from build123d import *

# Parameters (mm, degrees)
PAD003_DEPTH         = 6.35
SKETCH015_R          = 1.524
POCKET003_DEPTH      = 4.7635
POCKET003_DEPTH_BACK = 1.5885
SKETCH016_W          = 3.175
SKETCH016_H          = 12.7
PAD008_DEPTH         = 67.7
SKETCH025_W          = 28.575
SKETCH025_H          = 24.775
PAD009_DEPTH         = 3.175
POCKET007_DEPTH      = 5.175996
PAD010_DEPTH         = 3.175
CHAMFER001_SIZE      = 3.1496


with BuildPart() as part:
    # Sketch014 → Pad003 (new body, symmetric)
    with BuildSketch(Plane.YZ.offset(15.25)):
        with BuildLine():
            ThreePointArc((-1.430625, 0), (0.315625, -1.74625), (2.061875, 0))
            Line((2.061875, 5.63), (2.061875, 0))
            ThreePointArc((3.490625, 4.20125), (3.072154, 5.211529), (2.061875, 5.63))
            Line((3.490625, 4.20125), (3.490625, 0))
            ThreePointArc((0.315625, -3.175), (2.560689, -2.245064), (3.490625, 0))
            Line((-2.859375, -3.175), (0.315625, -3.175))
            Line((-2.859375, 4.20125), (-2.859375, -3.175))
            ThreePointArc((-1.430625, 5.63), (-2.440904, 5.211529), (-2.859375, 4.20125))
            Line((-1.430625, 5.63), (-1.430625, 0))
        make_face()
    extrude(amount=PAD003_DEPTH, both=True)

    # Sketch015 (on Face72 of LinearPattern001) → Pocket003 (cut, two sides)
    with BuildSketch(Plane.XZ.offset(1.271875)) as pocket003_sk:
        with Locations((12.075, 2.815)):
            Circle(SKETCH015_R)
        with Locations((18.425, 2.815)):
            Circle(SKETCH015_R)
    extrude(amount=-POCKET003_DEPTH, mode=Mode.SUBTRACT)
    extrude(pocket003_sk.sketch, amount=POCKET003_DEPTH_BACK, mode=Mode.SUBTRACT)

    # Sketch016 (on Face8 of Pocket003) → Pad008 (join)
    with BuildSketch(Plane(origin=(15.25, -2.859375, 0), x_dir=(0, 0, -1), z_dir=(0, -1, 0))):
        with Locations((1.5875, 0)):
            Rectangle(SKETCH016_W, SKETCH016_H)
    extrude(amount=PAD008_DEPTH)

    # Sketch025 (on Face16 of Pad008) → Pad009 (join)
    with BuildSketch(Plane(origin=(15.25, 0, 0), x_dir=(0, -1, 0), z_dir=(0, 0, 1))):
        with Locations((56.271875, -18.7375)):
            Rectangle(SKETCH025_W, SKETCH025_H)
    extrude(amount=-PAD009_DEPTH)

    # Sketch026 (on Face29 of Pad015) → Pocket007 (cut, through all)
    with BuildSketch(Plane(origin=(15.25, 0, 1.999996), x_dir=(0, -1, 0), z_dir=(0, 0, 1))):
        with BuildLine():
            ThreePointArc((61.161375, -8.9), (57.859375, -5.598), (54.557375, -8.9))
            Line((54.557375, -8.9), (54.557375, -21.6))
            ThreePointArc((54.557375, -21.6), (57.859375, -24.902), (61.161375, -21.6))
            Line((61.161375, -21.6), (61.161375, -8.9))
        make_face()
    extrude(amount=-POCKET007_DEPTH, mode=Mode.SUBTRACT)

    # Sketch027 (on Face24 of Pocket007) → Pad010 (join)
    with BuildSketch(Plane(origin=(15.25, 0, -3.175), x_dir=(0, 1, 0), z_dir=(0, 0, -1))):
        Polygon((-2.859375, 6.35), (-45.159375, 6.35), (-45.159375, -31.125), (-41.984375, -31.125), (-41.984375, 3.175), (-2.859375, 3.175), align=None)
    extrude(amount=PAD010_DEPTH)

    # Chamfer001
    chamfer001_edges = [part.edges().sort_by_distance(p)[0] for p in [
        (20.0125, -2.859375, -6.35),
        (-15.875, -43.571875, -6.35),
    ]]
    chamfer(chamfer001_edges, length=CHAMFER001_SIZE)


solid = part.part
Part model, mm, in its own coordinate system. A direction names the side the tool comes from. Coordinates: 2 decimals unless noted, no trailing zeros. Loops run counter-clockwise (first coordinate to the right, second up) from the corner with the lowest first, then second, coordinate; pieces in that order, holes last. Notation, with made-up numbers: (-30, 65.5) -> (13, 65.5) arc R24 cw to (13, 82.5) -> close; hole circle Ø6 at (-21, 69). An arc over 180 degrees is marked (long way). Use a Markdown table: item, result. Add a question column.
Item 1: Band-saw the part on A-A on x = -4.5. Write the cut outline in (y, z) (3 decimals).
Item 2: Probe probe 1 along Y at (x, z) = (-5, -2.5); probe 2 along Y at (x, z) = (-13.5, -0.5); probe 3 along X at (y, z) = (-60, -2.5) (3 decimals). List the from-to ranges inside material, lowest first.
Item 3: Which spindle directions (+Z, -Z, +X, -X, +Y, -Y) get a long thin tool onto all of the face, cutting with end or side? Do faces 5 (the flat face through (3, -52, -3.175)), 6 (the flat face through (15, 2.062, 3)), 7 (the flat face through (8.9, -17, -2)), 8 (the flat face through (0, -54.557, -2)), 9 (the flat face through (7, -44, 0)). Say none if no direction does.
Item 4: Band-saw the part on C-C on x = -12. Write the cut outline in (y, z) (3 decimals), plus the area to 3 significant figures.
Item 5: Pull direction Y, two halves, no side cores. Call faces 1 (the flat face through (15, -2.859, 2)), 2 (the flat face through (19.99, -4.41, -4.75)), 3 (the flat face through (14, -21, -3.175)), 4 (the flat face through (15, -1.431, 3)): +Y half, -Y half, draft (parallel to the pull), parting line (faces both ways), or undercut.
Item 6: Band-saw the part on B-B on z = -2.5. Write the cut outline in (x, y) (3 decimals).
Item 7: Flat gauge pins, fed straight in: P1, Ø3.5, axis at y = -24, z = -5, coming from the -X side (3 decimals); P2, Ø1, axis at x = 1.5, z = -1, coming from the +Y side; P3, Ø5, axis at x = 1, z = 1.5, coming from the -Y side; P4, Ø4.5, axis at y = -21, z = 0, coming from the -X side. Where does each tip first touch, or does it go through?
Geometry says:
| question | item | result |
|---|---|---|
| 1 | outline | (-70.559, -3.175) -> (-61.161, -3.175) -> (-61.161, 0) -> (-70.559, 0) -> close; (-54.557, -3.175) -> (-45.159, -3.175) -> (-45.159, -6.35) -> (-41.984, -6.35) -> (-41.984, 0) -> (-54.557, 0) -> close |
| 2 | probe 1 | -70.56 to -61.16, -54.56 to -41.98 |
| 2 | probe 2 | -70.56 to -41.98 |
| 2 | probe 3 | -15.875 to -8.864, 8.864 to 21.6 |
| 3 | face 5 | -Z, +X, -X, -Y |
| 3 | face 6 | +Z, +X, -X |
| 3 | face 7 | +Z, -Z, -X, +Y |
| 3 | face 8 | +Z, -Z |
| 3 | face 9 | +Z, +X, -X, -Y |
| 4 | outline | (-70.559, -3.175) -> (-45.159, -3.175) -> (-45.159, -6.35) -> (-41.984, -6.35) -> (-41.984, 0) -> (-70.559, 0) -> close |
| 4 | area | 101 mm² |
| 5 | face 1 | -Y half |
| 5 | face 2 | +Y half |
| 5 | face 3 | draft |
| 5 | face 4 | undercut |
| 6 | outline | (-15.875, -70.559) -> (21.6, -70.559) -> (21.6, 2.273) -> (8.9, 2.273) -> (8.9, -41.984) -> (-15.875, -41.984) -> close; hole (-6.35, -61.161) -> (6.35, -61.161) arc R3.302 ccw to (6.35, -54.557) -> (-6.35, -54.557) arc R3.302 ccw to start |
| 7 | P1 | x = 18.425 |
| 7 | P2 | y = -41.98 |
| 7 | P3 | y = -70.56 |
| 7 | P4 | x = 8.9 |
